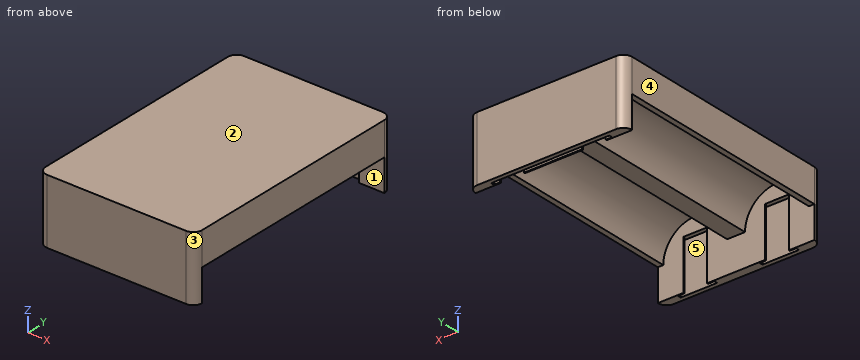
```python
from build123d import *

# Parameters (mm, degrees)
BOSS_EXTRUDE1_DEPTH  = 75
BOSS_EXTRUDE2_START  = -3
SKETCH1_3_R          = 10.75
BOSS_EXTRUDE2_DEPTH  = 3
CUT_EXTRUDE1_DEPTH   = 16.75
MIRROR3_COPY_1_DEPTH = 16.75
SKETCH5_W            = 15.25
SKETCH5_H            = 1.1
CUT_EXTRUDE2_DEPTH   = 2
FILLET1_R            = 3


with BuildPart() as part:
    # Sketch1 → Boss-Extrude1 (new body)
    with BuildSketch(Plane(origin=(0, 0, 0), x_dir=(1, 0, 0), z_dir=(0, 1, 0))):
        with BuildLine():
            Line((0, 0), (12.6, 0))
            Line((12.6, 0), (12.6, 0.4))
            ThreePointArc((12.6, 0.4), (4.998602102, 3.548602102), (1.85, 11.15))
            Line((1.85, 11.15), (0, 11.15))
            Line((0, 11.15), (0, 0))
        make_face()
        with BuildLine():
            Line((12.6, 0), (26.35, 0))
            Line((26.35, 0), (26.35, 11.15))
            Line((26.35, 11.15), (23.35, 11.15))
            ThreePointArc((23.35, 11.15), (20.201397898, 3.548602102), (12.6, 0.4))
            Line((12.6, 0.4), (12.6, 0))
        make_face()
        with BuildLine():
            Line((26.35, 11.15), (26.35, 0))
            Line((26.35, 0), (52.7, 0))
            Line((52.7, 0), (52.7, 11.15))
            Line((52.7, 11.15), (50.85, 11.15))
            ThreePointArc((50.85, 11.15), (40.1, 0.4), (29.35, 11.15))
            Line((29.35, 11.15), (26.35, 11.15))
        make_face()
    extrude(amount=BOSS_EXTRUDE1_DEPTH)

    # Sketch1<3> → Boss-Extrude2 (add)
    with BuildSketch(Plane(origin=(0, 0, 0), x_dir=(1, 0, 0), z_dir=(0, 1, 0)).offset(BOSS_EXTRUDE2_START)):
        with BuildLine():
            Line((50.85, 11.15), (52.7, 11.15))
            Line((52.7, 11.15), (52.7, 21.9))
            Line((52.7, 21.9), (40.1, 21.9))
            ThreePointArc((40.1, 21.9), (47.701397898, 18.751397898), (50.85, 11.15))
        make_face()
        with BuildLine():
            Line((26.35, 11.15), (26.35, 0))
            Line((26.35, 0), (52.7, 0))
            Line((52.7, 0), (52.7, 11.15))
            Line((52.7, 11.15), (50.85, 11.15))
            ThreePointArc((50.85, 11.15), (40.1, 0.4), (29.35, 11.15))
            Line((29.35, 11.15), (26.35, 11.15))
        make_face()
        with Locations((40.1, 11.15)):
            Circle(SKETCH1_3_R)
        with BuildLine():
            Line((23.35, 11.15), (26.35, 11.15))
            Line((26.35, 11.15), (29.35, 11.15))
            ThreePointArc((29.35, 11.15), (32.498602102, 18.751397898), (40.1, 21.9))
            Line((40.1, 21.9), (12.6, 21.9))
            ThreePointArc((12.6, 21.9), (20.201397898, 18.751397898), (23.35, 11.15))
        make_face()
        with BuildLine():
            Line((12.6, 0), (26.35, 0))
            Line((26.35, 0), (26.35, 11.15))
            Line((26.35, 11.15), (23.35, 11.15))
            ThreePointArc((23.35, 11.15), (20.201397898, 3.548602102), (12.6, 0.4))
            Line((12.6, 0.4), (12.6, 0))
        make_face()
        with Locations((12.6, 11.15)):
            Circle(SKETCH1_3_R)
        with BuildLine():
            Line((0, 0), (12.6, 0))
            Line((12.6, 0), (12.6, 0.4))
            ThreePointArc((12.6, 0.4), (4.998602102, 3.548602102), (1.85, 11.15))
            Line((1.85, 11.15), (0, 11.15))
            Line((0, 11.15), (0, 0))
        make_face()
        with BuildLine():
            ThreePointArc((1.85, 11.15), (4.998602102, 18.751397898), (12.6, 21.9))
            Line((12.6, 21.9), (0, 21.9))
            Line((0, 21.9), (0, 11.15))
            Line((0, 11.15), (1.85, 11.15))
        make_face()
    boss_extrude2 = extrude(amount=BOSS_EXTRUDE2_DEPTH)

    # Sketch4 → Cut-Extrude1 (cut)
    with BuildSketch(Plane(origin=(0, 0, -21.9), x_dir=(-1, 0, 0), z_dir=(0, 0, -1))):
        Polygon((-18.725, -1.5), (-6.475, -1.5), (-6.475, -0.4), (-8.6, -0.4), (-8.6, 0), (-16.6, 0), (-16.6, -0.4), (-18.725, -0.4), align=None)
    cut_extrude1 = extrude(amount=-CUT_EXTRUDE1_DEPTH, mode=Mode.SUBTRACT)

    # Mirror2: Cut-Extrude1 across plane
    add(cut_extrude1.mirror(Plane(origin=(26.35, 0, 0), x_dir=(0, 0, 1), z_dir=(1, 0, 0))), mode=Mode.SUBTRACT)

    # Mirror3: Boss-Extrude2, Cut-Extrude1 across plane
    add(boss_extrude2.mirror(Plane.ZX.offset(37.5)))
    add(cut_extrude1.mirror(Plane.ZX.offset(37.5)), mode=Mode.SUBTRACT)

    # Mirror3 copy 1 sketch → Mirror3 copy 1 (cut)
    with BuildSketch(Plane(origin=(52.7, 75, -21.9), x_dir=(1, 0, 0), z_dir=(0, 0, -1))):
        Polygon((-18.725, -1.5), (-6.475, -1.5), (-6.475, -0.4), (-8.6, -0.4), (-8.6, 0), (-16.6, 0), (-16.6, -0.4), (-18.725, -0.4), align=None)
    extrude(amount=-MIRROR3_COPY_1_DEPTH, mode=Mode.SUBTRACT)

    # Sketch5 → Cut-Extrude2 (cut)
    with BuildSketch(Plane(origin=(0, 0, -21.9), x_dir=(-1, 0, 0), z_dir=(0, 0, -1))):
        with Locations((-26.35, 75.95)):
            Rectangle(SKETCH5_W, SKETCH5_H)
    extrude(amount=-CUT_EXTRUDE2_DEPTH, mode=Mode.SUBTRACT)

    # Fillet1
    fillet1_edges = [part.edges().sort_by_distance(p)[0] for p in [
        (0, 78, -10.95),
        (52.7, 78, -10.95),
        (52.7, -3, -10.95),
        (0, -3, -10.95),
    ]]
    fillet(fillet1_edges, radius=FILLET1_R - 0.0001)  # a hair under: the kernel refuses the full size


solid = part.part
```
Input: part model. Units: mm. Frame: model coordinates. Face numbers are marked on the shaded views. A direction names the side the tool comes from. Coordinates: 2 decimals unless noted, no trailing zeros. Write each loop counter-clockwise with the first axis right and the second up, starting at its lowest first coordinate (ties: lowest second). Pieces come first, ordered by that corner, then holes. Notation, with made-up numbers: (3, -17.75) - (45, -17.75) arc R27 ccw to (45, 11.25) - close; hole circle Ø9 at (-31, 13). An arc over 180 degrees is marked (long way). Put each result on its own line as item: value. Start each with the question number.
1) Cut plane B-B (z = -1.5). Return the cut outline in (x, y).
2) Mould query, pull axis X, two halves, no side actions, for the marked faces 3, 4 and 5. Classes: pulls with the +X half, pulls with the -X half, needs draft (parallel to the pull), parting line crosses it, or undercut.
3) Cut plane A-A (x = 40.1). Return the cut outline in (y, z).
4) Ray query, L1, parallel to Y at x = 35, z = -14; L2, parallel to Y at x = 25, z = -13; L3, parallel to Y at x = 13.5, z = -9. Return the intervals inside material, ascending.
5) Cut plane D-D (x = 25.5). Return the cut outline in (y, z).
6) Reachability of the marked faces 1 and 2 from +Z, -Z, +X, -X, +Y, -Y: full face, straight path, thin tool, end or side. Return the list, or none.
7) Cut plane C-C (y = 10.5). Return the cut outline in (x, z), plus the area to 3 significant figures.
8) Contact query for flat-ended pins moving along their axis: pin 1 (0.5 mm diameter, centred on y = 75.5, z = -11.5, fed in from +X); pin 2 (1.6 mm diameter, centred on x = 15, y = -0.5, fed in from -Z); pin 3 (0.6 mm diameter, centred on y = -1, z = -10, fed in from -X); pin 4 (10 mm diameter, centred on x = 14, y = 50.5, fed in from +Z). Output: stop coordinate, or through.
Resolved:
1. outline: (0, 0) arc R3 ccw to (3, -3) - (49.7, -3) arc R3 ccw to (52.7, 0) - (52.7, 75) arc R3 ccw to (49.7, 78) - (3, 78) arc R3 ccw to (0, 75) - close; hole (7.86, 0) - (17.34, 0) - (17.34, 75) - (7.86, 75) - close; hole (35.36, 0) - (44.84, 0) - (44.84, 75) - (35.36, 75) - close
2. face 3: pulls with the +X half
2. face 4: pulls with the -X half
2. face 5: undercut
3. outline: (-3, -21.9) - (-1.5, -21.9) - (-1.5, -5.15) - (0, -5.15) - (0, -0.4) - (75, -0.4) - (75, -5.15) - (76.5, -5.15) - (76.5, -21.9) - (78, -21.9) - (78, 0) - (-3, 0) - close
4. L1: y = -3 to -1.5, -0.4 to 0, 75 to 75.4, 76.5 to 78
4. L2: y = -3 to 0, 75 to 78
4. L3: y = -3 to -1.5, 76.5 to 78
5. outline: (-3, -21.9) - (0, -21.9) - (0, -11.15) - (75, -11.15) - (75, -21.9) - (75.4, -21.9) - (75.4, -19.9) - (76.5, -19.9) - (76.5, -21.9) - (78, -21.9) - (78, 0) - (-3, 0) - close
6. face 1: -Z
6. face 2: +Z, +X, -X, +Y, -Y
7. outline: (0, -11.15) - (1.85, -11.15) arc R10.75 cw to (23.35, -11.15) - (29.35, -11.15) arc R10.75 cw to (50.85, -11.15) - (52.7, -11.15) - (52.7, 0) - (0, 0) - close
7. area: 225 mm2
8. pin 1: stops at x = 52.69
8. pin 2: stops at z = -5.15
8. pin 3: stops at x = 0.08
8. pin 4: stops at z = 0
